Read the model definition and answer for the solid it produces. Units are mm, in the model's axes. Give positions to 0.01 mm unless a question says otherwise; leave off trailing zeros. Loops run counter-clockwise (first coordinate to the right, second up) from the corner with the lowest first, then second, coordinate; pieces in that order, holes last. Notation, with made-up numbers: (-23.5, -20) - (-14.5, -20) arc R32 ccw to (-14.5, 17) - close; hole circle Ø4 at (19.5, -8.75). An arc over 180 degrees is marked (long way). Write each question's results on one line, items separated by ' | '. Start each with the question number.
Q1. The part is cut by section A-A, the plane y = -5.5. Write down the section's boundary in (x, z), plus the area to 3 significant figures.
Q2. The part is cut by section B-B, the plane x = -1. Write down the section's boundary in (y, z).
Q3. Given pin 1 (1.5 mm diameter, centred on x = 2, y = -3, fed in from -Z); pin 2 (0.5 mm diameter, centred on x = -0.5, z = -5.5, fed in from -Y); pin 3 (0.5 mm diameter, centred on y = 0.5, z = -5.5, fed in from -X); pin 4 (7.5 mm diameter, centred on x = 0, y = -2.5, fed in from +Z), each flat-ended and moving along its own axis, determine where each tip first touches the part or whether it passes through.
Q4. The part is cut by section C-C, the plane z = -6.75. Write down the section's boundary in (x, y), plus the area to 3 significant figures.
Q5. Find the intervals of material crossed by line 1 (Z direction, x = 2.75, y = -4.75); line 2 (Y direction, x = 1.5, z = -5.75), in increasing order. Write a range as from..to.
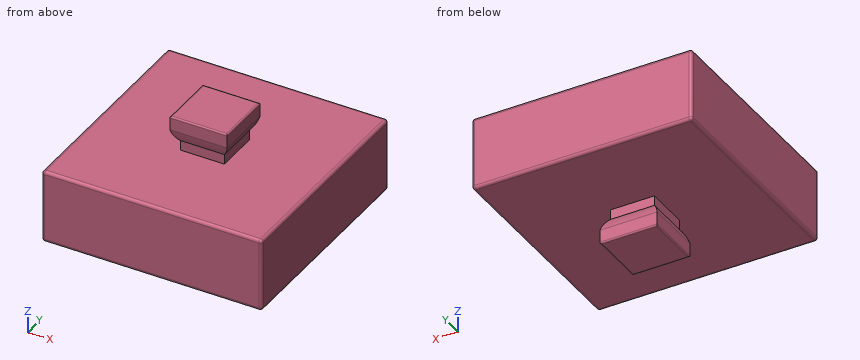
```python
from build123d import *

# Parameters (mm, degrees)
SKETCH_1_W                      = 15
SKETCH_1_H                      = 15
EXTRUDE_1_DEPTH                 = 5
SKETCH_2_W                      = 3
SKETCH_2_H                      = 3
EXTRUDE_2_DEPTH                 = 1
EXTRUDE_3_DEPTH                 = 2
CUT_EXTRUDE_1_REACH             = 13.726
CUT_EXTRUDE_1_DIRECTION_2_REACH = 13.726
FILLET_1_R                      = 0.1
FILLET_1_OF_MIRROR_1_R          = 0.1
FILLET_2_R                      = 0.2


with BuildPart() as part:
    # Sketch 1 → Extrude 1 (new body)
    with BuildSketch(Plane.XY):
        Rectangle(SKETCH_1_W, SKETCH_1_H)
    extrude(amount=-EXTRUDE_1_DEPTH)

    # Sketch 2 → Extrude 2 (add)
    with BuildSketch(Plane.XY):
        Rectangle(SKETCH_2_W, SKETCH_2_H)
    extrude_2 = extrude(amount=EXTRUDE_2_DEPTH)

    # Sketch 3 → Extrude 3 (add, symmetric)
    with BuildSketch(Plane(origin=(0, 0, 0), x_dir=(1, 0, 0), z_dir=(0, 1, 0))):
        with BuildLine():
            Line((-1.95, -2.5), (1.95, -2.5))
            Line((1.95, -2.5), (1.95, -1.555590279))
            ThreePointArc((1.95, -1.555590279), (1.780042303, -1.088161527), (1.5, -0.677124344))
            Line((1.5, -0.677124344), (-1.5, -0.677124344))
            ThreePointArc((-1.5, -0.677124344), (-1.780042303, -1.088161527), (-1.95, -1.555590279))
            Line((-1.95, -1.555590279), (-1.95, -2.5))
        make_face()
    extrude_3 = extrude(amount=EXTRUDE_3_DEPTH, both=True)

    # Sketch 4 → Cut-Extrude 1 (cut, up to next)
    with BuildSketch(Plane(origin=(0, 0, 0), x_dir=(0, 0, -1), z_dir=(1, 0, 0)), mode=Mode.PRIVATE) as cut_extrude_1_sk1:
        with BuildLine():
            Line((-2.5, 1.95), (-1.555590279, 1.95))
            ThreePointArc((-1.555590279, 1.95), (-1.088161527, 1.780042303), (-0.677124344, 1.5))
            Line((-0.677124344, 1.5), (-0.677124344, 2))
            Line((-0.677124344, 2), (-2.5, 2))
            Line((-2.5, 2), (-2.5, 1.95))
        make_face()
    cut_extrude_1_tool1 = extrude(cut_extrude_1_sk1.sketch, amount=-CUT_EXTRUDE_1_REACH, mode=Mode.PRIVATE) & part.part
    # Sketch 4 → Cut-Extrude 1 (cut, up to next)
    with BuildSketch(Plane(origin=(0, 0, 0), x_dir=(0, 0, -1), z_dir=(1, 0, 0)), mode=Mode.PRIVATE) as cut_extrude_1_sk2:
        with BuildLine():
            Line((-2.5, -2), (-0.677124344, -2))
            Line((-0.677124344, -2), (-0.677124344, -1.5))
            ThreePointArc((-0.677124344, -1.5), (-1.088161527, -1.780042303), (-1.555590279, -1.95))
            Line((-1.555590279, -1.95), (-2.5, -1.95))
            Line((-2.5, -1.95), (-2.5, -2))
        make_face()
    cut_extrude_1_tool2 = extrude(cut_extrude_1_sk2.sketch, amount=-CUT_EXTRUDE_1_REACH, mode=Mode.PRIVATE) & part.part
    cut_extrude_1_1 = cut_extrude_1_tool1.solids().sort_by_distance((0, 1.873038, 1.175075))[0]
    add(cut_extrude_1_1, mode=Mode.SUBTRACT)
    cut_extrude_1_2 = cut_extrude_1_tool2.solids().sort_by_distance((0, -1.873038, 1.175075))[0]
    add(cut_extrude_1_2, mode=Mode.SUBTRACT)
    cut_extrude_1 = cut_extrude_1_1 + cut_extrude_1_2  # Cut-Extrude 1 as one shape, for the pattern or mirror that repeats it

    # Sketch 4 → Cut-Extrude 1 direction 2 (cut, up to next)
    with BuildSketch(Plane(origin=(0, 0, 0), x_dir=(0, 0, -1), z_dir=(1, 0, 0)), mode=Mode.PRIVATE) as cut_extrude_1_direction_2_sk1:
        with BuildLine():
            Line((-2.5, 1.95), (-1.555590279, 1.95))
            ThreePointArc((-1.555590279, 1.95), (-1.088161527, 1.780042303), (-0.677124344, 1.5))
            Line((-0.677124344, 1.5), (-0.677124344, 2))
            Line((-0.677124344, 2), (-2.5, 2))
            Line((-2.5, 2), (-2.5, 1.95))
        make_face()
    cut_extrude_1_direction_2_tool1 = extrude(cut_extrude_1_direction_2_sk1.sketch, amount=CUT_EXTRUDE_1_DIRECTION_2_REACH, mode=Mode.PRIVATE) & part.part
    # Sketch 4 → Cut-Extrude 1 direction 2 (cut, up to next)
    with BuildSketch(Plane(origin=(0, 0, 0), x_dir=(0, 0, -1), z_dir=(1, 0, 0)), mode=Mode.PRIVATE) as cut_extrude_1_direction_2_sk2:
        with BuildLine():
            Line((-2.5, -2), (-0.677124344, -2))
            Line((-0.677124344, -2), (-0.677124344, -1.5))
            ThreePointArc((-0.677124344, -1.5), (-1.088161527, -1.780042303), (-1.555590279, -1.95))
            Line((-1.555590279, -1.95), (-2.5, -1.95))
            Line((-2.5, -1.95), (-2.5, -2))
        make_face()
    cut_extrude_1_direction_2_tool2 = extrude(cut_extrude_1_direction_2_sk2.sketch, amount=CUT_EXTRUDE_1_DIRECTION_2_REACH, mode=Mode.PRIVATE) & part.part
    cut_extrude_1_direction_2_1 = cut_extrude_1_direction_2_tool1.solids().sort_by_distance((0, 1.873038, 1.175075))[0]
    add(cut_extrude_1_direction_2_1, mode=Mode.SUBTRACT)
    cut_extrude_1_direction_2_2 = cut_extrude_1_direction_2_tool2.solids().sort_by_distance((0, -1.873038, 1.175075))[0]
    add(cut_extrude_1_direction_2_2, mode=Mode.SUBTRACT)
    cut_extrude_1_direction_2 = cut_extrude_1_direction_2_1 + cut_extrude_1_direction_2_2  # Cut-Extrude 1 direction 2 as one shape, for the pattern or mirror that repeats it

    # Fillet 1
    fillet_1_edges = [part.edges().sort_by_distance(p)[0] for p in [
        (-1.95, 0, 2.5),
        (1.95, 0, 2.5),
        (0, -1.95, 2.5),
        (0, 1.95, 2.5),
    ]]
    fillet(fillet_1_edges, radius=FILLET_1_R)

    # Mirror 1: Extrude 2, Extrude 3, Cut-Extrude 1, Cut-Extrude 1 direction 2 across plane
    add(extrude_2.mirror(Plane.XY.offset(-2.5)))
    add(extrude_3.mirror(Plane.XY.offset(-2.5)))
    add(cut_extrude_1.mirror(Plane.XY.offset(-2.5)), mode=Mode.SUBTRACT)
    add(cut_extrude_1_direction_2.mirror(Plane.XY.offset(-2.5)), mode=Mode.SUBTRACT)

    # Fillet 1 of Mirror 1
    fillet_1_of_mirror_1_edges = [part.edges().sort_by_distance(p)[0] for p in [
        (-1.95, 0, -7.5),
        (1.95, 0, -7.5),
        (0, -1.95, -7.5),
        (0, 1.95, -7.5),
    ]]
    fillet(fillet_1_of_mirror_1_edges, radius=FILLET_1_OF_MIRROR_1_R)

    # Fillet 2
    fillet_2_edges = [part.edges().sort_by_distance(p)[0] for p in [
        (7.5, 0, -5),
        (0, 7.5, -5),
        (-7.5, 0, -5),
        (0, 7.5, 0),
        (7.5, 0, 0),
        (0, -7.5, 0),
        (-7.5, 0, 0),
        (0, -7.5, -5),
        (-7.5, 7.5, -2.5),
        (7.5, 7.5, -2.5),
        (7.5, -7.5, -2.5),
        (-7.5, -7.5, -2.5),
    ]]
    fillet(fillet_2_edges, radius=FILLET_2_R)


solid = part.part
```
Check sheet entries:
1) outline: (-7.5, -4.8) arc R0.2 ccw to (-7.3, -5) - (7.3, -5) arc R0.2 ccw to (7.5, -4.8) - (7.5, -0.2) arc R0.2 ccw to (7.3, 0) - (-7.3, 0) arc R0.2 ccw to (-7.5, -0.2) - close | area: 75.0 mm^2
2) outline: (-7.5, -4.8) arc R0.2 ccw to (-7.3, -5) - (-1.5, -5) - (-1.5, -5.68) arc R2 ccw to (-1.95, -6.56) - (-1.95, -7.4) arc R0.1 ccw to (-1.85, -7.5) - (1.85, -7.5) arc R0.1 ccw to (1.95, -7.4) - (1.95, -6.56) arc R2 ccw to (1.5, -5.68) - (1.5, -5) - (7.3, -5) arc R0.2 ccw to (7.5, -4.8) - (7.5, -0.2) arc R0.2 ccw to (7.3, 0) - (1.5, 0) - (1.5, 0.68) arc R2 ccw to (1.95, 1.56) - (1.95, 2.4) arc R0.1 ccw to (1.85, 2.5) - (-1.85, 2.5) arc R0.1 ccw to (-1.95, 2.4) - (-1.95, 1.56) arc R2 ccw to (-1.5, 0.68) - (-1.5, 0) - (-7.3, 0) arc R0.2 ccw to (-7.5, -0.2) - close
3) pin 1: stops at z = -5 | pin 2: stops at y = -1.56 | pin 3: stops at x = -1.56 | pin 4: stops at z = 2.5
4) outline: (-1.95, -1.95) - (1.95, -1.95) - (1.95, 1.95) - (-1.95, 1.95) - close | area: 15.2 mm^2
5) line 1: z = -5..0 | line 2: y = -1.56..1.56
